Read the model definition and answer for the solid it produces. Units are mm, in the model's axes. A direction names the side the tool comes from. Coordinates: 2 decimals unless noted, no trailing zeros. Write each loop counter-clockwise with the first axis right and the second up, starting at its lowest first coordinate (ties: lowest second). Pieces come first, ordered by that corner, then holes. Notation, with made-up numbers: (39, 7.25) -> (56, 7.25) arc R7 ccw to (56, 13.25) -> close; hole circle Ø11 at (16, 32). An arc over 180 degrees is marked (long way). Return JSON: item names as keys, results as strings.
from build123d import *

# Parameters (mm, degrees)
EXTRUDE_1_DEPTH     = 250
CUT_EXTRUDE_1_DEPTH = 250


with BuildPart() as part:
    # Эскиз1 → Бобышка-Вытянуть1 (new body)
    with BuildSketch(Plane(origin=(0, 0, 0), x_dir=(1, 0, 0), z_dir=(0, 1, 0))):
        Polygon((0, 0), (0, 2), (20, 2), (20, 22), (22, 22), (22, 0), align=None)
    extrude(amount=EXTRUDE_1_DEPTH)

    # Эскиз3 → Вырез-Вытянуть1 (cut)
    with BuildSketch(Plane(origin=(22, 0, 0), x_dir=(0, 0, -1), z_dir=(1, 0, 0))):
        Polygon((0, 0), (22, 0), (22, 22), align=None)
        Polygon((22, 250), (22, 228), (0, 250), align=None)
    extrude(amount=-CUT_EXTRUDE_1_DEPTH, mode=Mode.SUBTRACT)


solid = part.part
1. The part is cut by section A-A (y = 17). Determine the outline of the cut face in (x, z), then the cut area to 3 significant figures.
Taken from the geometry:
{"outline": "(0, -2) -> (20, -2) -> (20, -17) -> (22, -17) -> (22, 0) -> (0, 0) -> close", "area": "74.0 mm2"}
2. The part is cut by section D-D (y = 190.5). Determine the outline of the cut face in (x, z).
Taken from the geometry:
{"outline": "(0, -2) -> (20, -2) -> (20, -22) -> (22, -22) -> (22, 0) -> (0, 0) -> close"}
3. The part is cut by section B-B (x = 16). Determine the outline of the cut face in (y, z), then the cut area to 3 significant figures.
Taken from the geometry:
{"outline": "(0, 0) -> (2, -2) -> (248, -2) -> (250, 0) -> close", "area": "496 mm2"}
4. Consider L1, parallel to X at y = 53, z = -2.75; L2, parallel to Z at x = 5, y = 183.5. Determine where each line is inside the solid, lowest interval first.
Taken from the geometry:
{"L1": "x = 20 to 22", "L2": "z = -2 to 0"}
5. The part is cut by section C-C (z = -15.25). Determine the outline of the cut face in (x, y).
Taken from the geometry:
{"outline": "(20, 15.25) -> (22, 15.25) -> (22, 234.75) -> (20, 234.75) -> close"}
6. A tool of negligible diameter and unlimited length cuts with its end or side. For faces 1 (the face through (10, 123, -2)), 2 (the face through (22, 123, -11)), from which of +Z, -Z, +X, -X, +Y, -Y can it reach the whole face along a straight path? Write none if from no direction.
Taken from the geometry:
{"face 1": "-Z, -X, +Y, -Y", "face 2": "+Z, -Z, +X, +Y, -Y"}
7. Flat-ended cylindrical pins translate along their axes: pin 1 Ø6 at (x, y) = (7.5, 196.5) entering from -Z; pin 2 Ø10 at (y, z) = (154, -8) entering from -X; pin 3 Ø2 at (x, z) = (7, -2.5) entering from -Y. Find the tip coordinate at first contact, or state that the pin passes through.
Taken from the geometry:
{"pin 1": "stops at z = -2", "pin 2": "stops at x = 20", "pin 3": "stops at y = 1.5"}
